from build123d import *

# Parameters (mm, degrees)
EXTRUDE_1_DEPTH        = 8
HOLE_WIZARD_M8_1_D     = 6.8
HOLE_WIZARD_M8_1_DEPTH = 19.75
HOLE_WIZARD_M8_1_TIP   = 2.042926105


with BuildPart() as part:
    # 草图1 → 凸台-拉伸1 (new, symmetric)
    with BuildSketch(Plane.XY):
        with BuildLine():
            Line((3.8, 0), (-3.8, 0))
            ThreePointArc((-3.8, 0), (-6.087496121, 1.207061519), (-7.85, 3.1))
            Line((-7.85, 3.1), (-7.85, 3.9))
            ThreePointArc((-7.85, 3.9), (-7.791421356, 4.041421356), (-7.65, 4.1))
            Line((-7.65, 4.1), (-4, 4.1))
            Line((-4, 4.1), (-4, 5.8))
            ThreePointArc((-4, 5.8), (-3.941421356, 5.941421356), (-3.8, 6))
            Line((-3.8, 6), (3.8, 6))
            ThreePointArc((3.8, 6), (3.941421356, 5.941421356), (4, 5.8))
            Line((4, 5.8), (4, 4.1))
            Line((4, 4.1), (7.65, 4.1))
            ThreePointArc((7.65, 4.1), (7.791421356, 4.041421356), (7.85, 3.9))
            Line((7.85, 3.9), (7.85, 3.1))
            ThreePointArc((7.85, 3.1), (6.087496121, 1.207061519), (3.8, 0))
        make_face()
    extrude(amount=EXTRUDE_1_DEPTH, both=True)

    # M8 螺纹孔1
    with Locations(Plane.ZX.offset(6)):
        with Locations((0, 0)):
            Hole(HOLE_WIZARD_M8_1_D / 2, depth=HOLE_WIZARD_M8_1_DEPTH)
            with Locations((0, 0, -(HOLE_WIZARD_M8_1_DEPTH + HOLE_WIZARD_M8_1_TIP / 2))):  # 118° drill point
                Cone(0, HOLE_WIZARD_M8_1_D / 2, HOLE_WIZARD_M8_1_TIP, mode=Mode.SUBTRACT)


solid = part.part
Can you work these out from the model? Positions are in its coordinate system, mm. A direction names the side the tool comes from. Coordinates: 2 decimals unless noted, no trailing zeros. Write each loop counter-clockwise with the first axis right and the second up, starting at its lowest first coordinate (ties: lowest second). Pieces come first, ordered by that corner, then holes. Notation, with made-up numbers: (-24.75, -19) - (30.25, -19) arc R17 ccw to (30.25, 4) - close; hole circle Ø3 at (53.5, 10.25). An arc over 180 degrees is marked (long way). Return JSON: item names as keys, results as strings. Group by question number.
Item 1: If we section it at B-B (x = 0): Write out the boundary of the cut face in (y, z), then the cut area to 3 significant figures.
Item 2: If we section it at D-D (z = 4.75): Write out the boundary of the cut face in (x, y), then the cut area to 3 significant figures.
Item 3: Please list where these lines run through material, in increasing order: probe 1 along X at (y, z) = (4.15, 0); probe 2 along Z at (x, y) = (3, 2.15); probe 3 along X at (y, z) = (3.05, -1.5).
Item 4: If we section it at A-A (z = 0): Write out the boundary of the cut face in (x, y).
Item 5: If we section it at C-C (y = 3.65): Write out the boundary of the cut face in (x, z), then the cut area to 3 significant figures.
Item 6: We'd pull the mould along X, two halves only. Please class faces 1 (the face through (0, 0, 4)), 2 (the face through (-3.32, 2.96, 0.74)), 3 (the face through (-4, 5, 0)): pulls with the +X half, pulls with the -X half, needs draft (parallel to the pull), parting line crosses it, or undercut.
Item 7: I'm going to push flat-ended pins straight in: pin 1 Ø1.1 at (x, z) = (-6.5, -0.5) entering from +Y; pin 2 Ø1.4 at (y, z) = (5, -3) entering from -X. Where does each tip first touch, or does it pass through?
Item 8: Which directions (+Z, -Z, +X, -X, +Y, -Y) give clear straight access to the entire face, cutting with the end or side of a thin tool? Please do faces 4 (the face through (-6, 4.1, 0)), 5 (the face through (6, 4.1, 0)), 6 (the face through (-7.85, 3.5, 0.1)).
Return value:
{
 "1": {"outline": "(0, -8) - (6, -8) - (6, -3.4) - (0, -3.4) - close; (0, 3.4) - (6, 3.4) - (6, 8) - (0, 8) - close", "area": "55.2 mm^2"},
 "2": {"outline": "(-7.85, 3.1) arc R7.74 ccw to (-3.8, 0) - (3.8, 0) arc R7.74 ccw to (7.85, 3.1) - (7.85, 3.9) arc R0.2 ccw to (7.65, 4.1) - (4, 4.1) - (4, 5.8) arc R0.2 ccw to (3.8, 6) - (-3.8, 6) arc R0.2 ccw to (-4, 5.8) - (-4, 4.1) - (-7.65, 4.1) arc R0.2 ccw to (-7.85, 3.9) - close", "area": "69.9 mm^2"},
 "3": {"probe 1": "x = -4 to -3.4, 3.4 to 4", "probe 2": "z = -8 to -1.6, 1.6 to 8", "probe 3": "x = -7.82 to -3.05, 3.05 to 7.82"},
 "4": {"outline": "(-7.85, 3.1) arc R7.74 ccw to (-3.8, 0) - (-3.4, 0) - (-3.4, 6) - (-3.8, 6) arc R0.2 ccw to (-4, 5.8) - (-4, 4.1) - (-7.65, 4.1) arc R0.2 ccw to (-7.85, 3.9) - close; (3.4, 0) - (3.8, 0) arc R7.74 ccw to (7.85, 3.1) - (7.85, 3.9) arc R0.2 ccw to (7.65, 4.1) - (4, 4.1) - (4, 5.8) arc R0.2 ccw to (3.8, 6) - (3.4, 6) - close"},
 "5": {"outline": "(-7.85, -8) - (7.85, -8) - (7.85, 8) - (-7.85, 8) - close; hole circle Ø6.8 at (0, 0)", "area": "215 mm^2"},
 "6": {"face 1": "needs draft", "face 2": "undercut", "face 3": "pulls with the -X half"},
 "7": {"pin 1": "stops at y = 4.1", "pin 2": "stops at x = -4"},
 "8": {"face 4": "+Z, -Z, -X, +Y", "face 5": "+Z, -Z, +X, +Y", "face 6": "+Z, -Z, -X, +Y, -Y"}
}
